```python
from build123d import *

# Parameters (mm, degrees)
F0_W     = 31.75
F0_H     = 31.75
F1_DEPTH = 508
F2_R     = 3.175
F3_T     = -3.048


with BuildPart() as f1:
    # F0 (on Top) → F1 (new body)
    with BuildSketch(Plane.XY):
        Rectangle(F0_W, F0_H)
    extrude(amount=-F1_DEPTH)

    # F2
    f2_edges = [f1.edges().sort_by_distance(p)[0] for p in [
        (-15.875, 15.875, -254),
        (-15.875, -15.875, -254),
        (15.875, 15.875, -254),
        (15.875, -15.875, -254),
    ]]
    fillet(f2_edges, radius=F2_R)

    # F3
    f3_openings = [f1.faces().sort_by_distance(p)[0] for p in [
        (0, 0, 0),
        (0, 0, -508),
    ]]
    offset(amount=F3_T, openings=f3_openings)


solid = f1.part
```
Geometry: final body of the model. Coordinates: model frame, mm. A direction names the side the tool comes from. Round coordinates to 2 decimals unless told otherwise and drop trailing zeros. Loops run counter-clockwise (first coordinate to the right, second up) from the corner with the lowest first, then second, coordinate; pieces in that order, holes last. Notation, with made-up numbers: (29, 0) -> (59, 0) arc R13 ccw to (59, 15) -> close; hole circle Ø3 at (15.5, 66). An arc over 180 degrees is marked (long way). Use one line per item in the form item = value. Start each with the question number.
1) First-contact query: P1, Ø10, axis at x = 9, y = -7, coming from the +Z side; P2, Ø12, axis at x = -0.5, y = 3, coming from the -Z side. Flat tips, straight axial feed; report the tip coordinate or a pass-through.
2) Line query: L1, parallel to X at y = 10, z = -304.5 (3 decimals); L2, parallel to X at y = -13, z = -418. Output: solid intervals per line, ascending.
3) Draft query along Y for faces 3 (the flat face through (0, 15.875, -250)), 4 (the flat face through (0, -12.827, -250)), 5 (the flat face through (-14, 0, 0)). Return one class per face: released by +Y, released by -Y, zero draft, split by the parting line, or undercut.
4) Section C-C on z = -112.5. Output: boundary loops of the cut face in (x, y) (3 decimals), then the cut area to 3 significant figures.
5) Access query for faces 1 (the flat face through (0, -15.875, -250)), 2 (the flat face through (-12.827, 0, -250)). Directions: +Z, -Z, +X, -X, +Y, -Y. A direction counts if a zero-diameter tool reaches every point of the face in a straight line with its end or side. Return the directions, or none.
6) Section A-A on x = 2. Output: boundary loops of the cut face in (y, z) (3 decimals).
Response:
q1.P1 = 0
q1.P2 = through
q2.L1 = -15.875 to -12.827, 12.827 to 15.875
q2.L2 = -15.86 to 15.86
q3.face_3 = released by +Y
q3.face_4 = undercut
q3.face_5 = zero draft
q4.outline = (-15.875, -12.7) arc R3.175 ccw to (-12.7, -15.875) -> (12.7, -15.875) arc R3.175 ccw to (15.875, -12.7) -> (15.875, 12.7) arc R3.175 ccw to (12.7, 15.875) -> (-12.7, 15.875) arc R3.175 ccw to (-15.875, 12.7) -> close; hole (-12.827, -12.7) arc R0.127 ccw to (-12.7, -12.827) -> (12.7, -12.827) arc R0.127 ccw to (12.827, -12.7) -> (12.827, 12.7) arc R0.127 ccw to (12.7, 12.827) -> (-12.7, 12.827) arc R0.127 ccw to (-12.827, 12.7) -> close
q4.area = 341 mm^2
q5.face_1 = +Z, -Z, +X, -X, -Y
q5.face_2 = +Z, -Z
q6.outline = (-15.875, -508) -> (-12.827, -508) -> (-12.827, 0) -> (-15.875, 0) -> close; (12.827, -508) -> (15.875, -508) -> (15.875, 0) -> (12.827, 0) -> close
